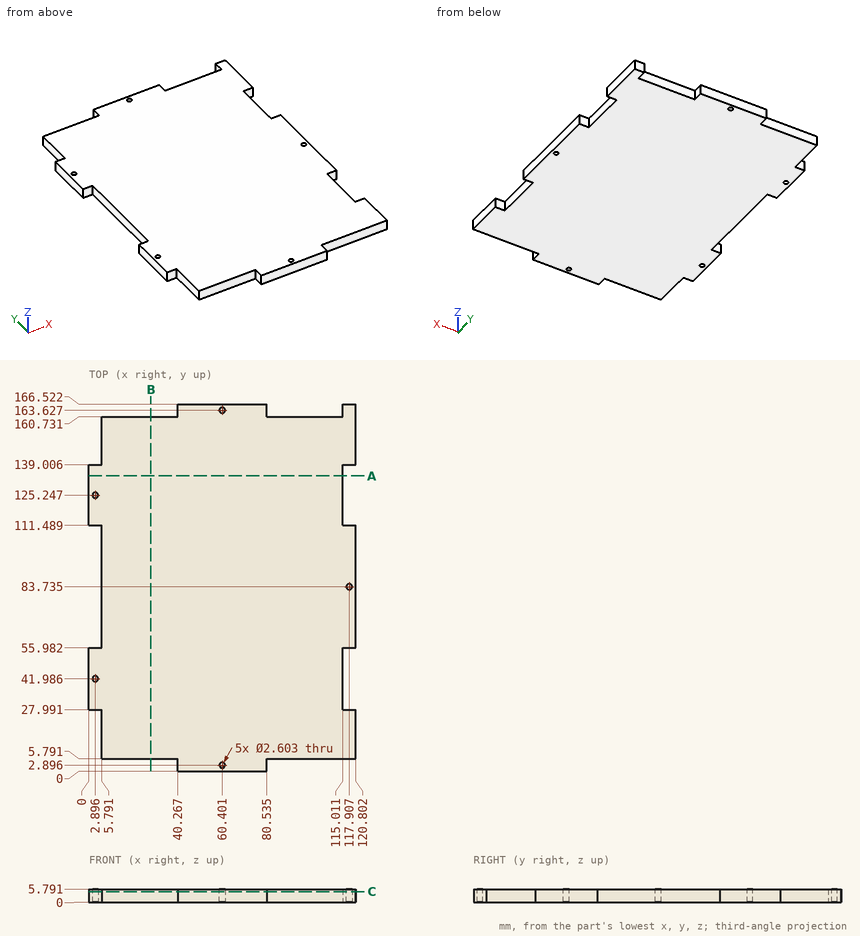
Print and shaded views of the part. All mm, measured from the part's lowest x, y and z. Coordinates: 2 decimals unless noted, no trailing zeros. Order: outer loops, then holes, each group sorted by start corner. A loop starts at its lowest first (then second) coordinate and runs counter-clockwise, first axis right, second up.
Item 1: Drop flat-ended pins along their axis: pin 1 Ø3.5 at (x, y) = (60.4, 2.9) entering from +Z; pin 2 Ø3 at (y, z) = (79, 0.5) entering from -X; pin 3 Ø3 at (x, z) = (3, 2) entering from -Y; pin 4 Ø1.7 at (x, z) = (2.5, 4) entering from +Y. Give the stop position or say it passes through.
Filled in:
pin 1: stops at z = 5.79
pin 2: stops at x = 5.79
pin 3: stops at y = 27.99
pin 4: stops at y = 139.01
Item 2: Saw through at A-A on y = 134. List the corners of the cut face in (x, z).
Filled in:
outline: (0, 0) - (115.01, 0) - (115.01, 5.79) - (0, 5.79) - close
Item 3: Saw through at B-B on x = 28. List the corners of the cut face in (y, z).
Filled in:
outline: (5.79, 0) - (160.73, 0) - (160.73, 5.79) - (5.79, 5.79) - close
Item 4: Drill centre lines: L1, parallel to X at y = 47, z = 4.2; L2, parallel to Y at x = 9, z = 4.55; L3, parallel to X at y = 7, z = 5.15. Where is each one in solid material? Low to high.
Filled in:
L1: x = 0 to 115.01
L2: y = 5.79 to 160.73
L3: x = 5.79 to 120.8
Item 5: Saw through at C-C on z = 4.75. State how many separate pieces and enclosed holes the cut face has, then the cut area to 3 significant figures.
Filled in:
separate pieces: 1
enclosed holes: 5
area: 18,300 mm2
